Geometry: final body of the model. Coordinates: model frame, mm. A direction names the side the tool comes from. Round coordinates to 2 decimals unless told otherwise and drop trailing zeros. Loops run counter-clockwise (first coordinate to the right, second up) from the corner with the lowest first, then second, coordinate; pieces in that order, holes last. Notation, with made-up numbers: M 70.25,20 L 126.25,20 A23 ccw 126.25,42 Z; hole C 52,27.5 d3. An arc over 180 degrees is marked long. Answer as a JSON object with one key per item and string values.
from build123d import *

# Parameters (mm, degrees)
M4_TAPPED_HOLE1_D           = 3.3
M4_TAPPED_HOLE1_CSINK_D     = 4.05
M4_TAPPED_HOLE1_CSINK_ANGLE = 90
FILLET3_R                   = 0.5
CHAMFER1_SIZE               = 0.1


with BuildPart() as part:
    # Sketch2 → Revolve1 (revolve)
    with BuildSketch(Plane.XY, mode=Mode.PRIVATE) as revolve1_sk:
        Polygon((-24.382296362, 0), (-17.415327427, 0), (-16.082296362, 0), (-16.082296362, 2.15), (-13.382296362, 2.15), (-13.382296362, 3.3), (-14.042296362, 3.3), (-14.042296362, 3.15), (-17.192296362, 3.15), (-17.762296362, 2.58), (-19.382296362, 2.58), (-21.082296362, 3.196283143), (-22.082296362, 3.196283143), (-24.382296362, 2.58), align=None)
    revolve(revolve1_sk.sketch.rotate(Axis((-24.382296362, 0, 0), (1, 0, 0)), 90), axis=Axis((-24.382296362, 0, 0), (1, 0, 0)))

    # M4 Tapped Hole1 (through all)
    with Locations(Plane.ZY.offset(24.382296362)):
        with Locations((0, 0)):
            CounterSinkHole(M4_TAPPED_HOLE1_D / 2, M4_TAPPED_HOLE1_CSINK_D / 2, counter_sink_angle=M4_TAPPED_HOLE1_CSINK_ANGLE)

    # Fillet3
    fillet3_edges = [part.edges().sort_by_distance(p)[0] for p in [
        (-24.382296362, 0, -2.58),
    ]]
    fillet(fillet3_edges, radius=FILLET3_R)

    # Chamfer1
    chamfer1_edges = [part.edges().sort_by_distance(p)[0] for p in [
        (-13.382296362, 0, -2.15),
        (-13.382296362, 0, -3.3),
        (-14.042296362, 0, -3.15),
    ]]
    chamfer(chamfer1_edges, length=CHAMFER1_SIZE)


solid = part.part
1) Ray query, line 1 (Y direction, x = -14.2, z = 0); line 2 (Y direction, x = -16.25, z = -1.25); line 3 (Z direction, x = -18.75, y = -0.75). Return the intervals inside material, ascending.
Results:
{"line 1": "-3.15 to -2.15, 2.15 to 3.15", "line 2": "-2.89 to -1.08, 1.08 to 2.89", "line 3": "-2.47 to -1.47, 1.47 to 2.47"}
2) Section query A-A (x = -16.25). Return the cut outline in (y, z).
Results:
{"outline": "C 0,0 d6.3; hole C 0,0 d3.3"}
3) Reachability of faces 1 (the cylindrical face through (-21.59, -3.17, -0.42)), 2 (the cylindrical face through (-15.689, 1.917, -2.5)) from +Z, -Z, +X, -X, +Y, -Y: full face, straight path, thin tool, end or side. Return the list, or none.
Results:
{"face 1": "-X", "face 2": "none"}
4) Pull-direction query (Z, two-part tool) for faces 3 (the cylindrical face through (-19.989, 1.115, 1.216)), 4 (the flat face through (-13.382, 2.1, -1.4)), 5 (the cylindrical face through (-14.76, -0.09, -2.15)), 6 (the cylindrical face through (-13.77, -2.23, -2.43)); classes: +Z half, -Z half, draft (parallel to the pull), parting line (faces both ways), or undercut.
Results:
{"face 3": "undercut", "face 4": "draft", "face 5": "undercut", "face 6": "parting line"}
5) Pin query (flat end, axial travel): P1, Ø2, axis at y = -1, z = 0.5, coming from the +X side; P2, Ø1, axis at x = -23, y = 0.5, coming from the -Z side. Return the tip coordinate at first contact, or that it passes through.
Results:
{"P1": "x = -16.08", "P2": "z = -3.06"}
6) Section query B-B (x = -15). Return the cut outline in (y, z).
Results:
{"outline": "C 0,0 d6.3; hole C 0,0 d4.3"}
